For this review, take the finished solid that the model builds, in its own axes (mm). A direction names the side the tool comes from. Round coordinates to 2 decimals unless told otherwise and drop trailing zeros. Order: outer loops, then holes, each group sorted by start corner. A loop starts at its lowest first (then second) coordinate and runs counter-clockwise, first axis right, second up. Notation, with made-up numbers: M -33.5,-14.75 L 0.5,-14.75 A12 cw 0.5,2.25 Z; hole C 5.25,26.25 d7. An arc over 180 degrees is marked long. Answer as a JSON object with one key per item and string values.
from build123d import *

# Parameters (mm, degrees)
F0_W     = 12.7
F0_H     = 25.4
F1_DEPTH = 25.4
F3_DEPTH = 6.35
F5_D     = 6.35
F7_D     = 6.35


with BuildPart() as f1:
    # F0 (on Top) → F1 (new body)
    with BuildSketch(Plane.XY):
        with Locations((-6.35, 12.7)):
            Rectangle(F0_W, F0_H)
    extrude(amount=F1_DEPTH)

    # F2 (on Top) → F3 (join)
    with BuildSketch(Plane.XY):
        with BuildLine():
            Line((0, 25.4), (0, 0))
            Line((0, 0), (12.7, 0))
            ThreePointArc((12.7, 0), (25.4, 12.7), (12.7, 25.4))
            Line((12.7, 25.4), (0, 25.4))
        make_face()
    extrude(amount=F3_DEPTH)

    # F5 (through all)
    with Locations(Plane.YZ):
        with Locations((12.7, 15.875)):
            Hole(F5_D / 2)

    # F7 (through all)
    with Locations(Plane.XY.offset(6.35)):
        with Locations((12.7, 12.7)):
            Hole(F7_D / 2)


solid = f1.part
1) Add section B-B on x = -5. State the section outline as (y, z) points (3 decimals).
Geometry check:
{"outline": "M 0,0 L 25.4,0 L 25.4,25.4 L 0,25.4 Z; hole C 12.7,15.875 d6.35"}
2) Add section D-D on z = 15. State the section outline as (x, y) points.
Geometry check:
{"outline": "M -12.7,0 L 0,0 L 0,9.65 L -12.7,9.65 Z; M -12.7,15.75 L 0,15.75 L 0,25.4 L -12.7,25.4 Z"}
3) Add section C-C on z = 3.25. State the section outline as (x, y) points (3 decimals), and give its area (3 significant figures).
Geometry check:
{"outline": "M -12.7,0 L 12.7,0 A12.7 ccw 12.7,25.4 L -12.7,25.4 Z; hole C 12.7,12.7 d6.35", "area": "867 mm²"}
4) For L1, parallel to Z at x = -7.5, y = 12.7; L2, parallel to Y at x = 12.7, z = 2 (3 decimals); L3, parallel to X at y = 18, z = 24, list the stretches that pass through material, from the lowest coordinate up.
Geometry check:
{"L1": "z = 0 to 12.7, 19.05 to 25.4", "L2": "y = 0 to 9.525, 15.875 to 25.4", "L3": "x = -12.7 to 0"}
5) Mouldability with a two-part tool opening along Y and no side actions: class faces 3 (the cylindrical face through (-6.44, 9.67, 16.83)), 4 (the flat face through (-5, 25.4, 10)), 5 (the flat face through (6, 13, 0)) as +Y half, -Y half, draft (parallel to the pull), parting line (faces both ways), or undercut.
Geometry check:
{"face 3": "undercut", "face 4": "+Y half", "face 5": "draft"}
6) Insertion check: P1, Ø6, axis at y = 8.5, z = 14.5, coming from the +X side; P2, Ø4, axis at x = 12.7, y = 12.7, coming from the -Z side; P3, Ø4, axis at x = 10.5, y = 20, coming from the -Z side; P4, Ø2, axis at x = 6.5, y = 18, coming from the +Z side. Each pin has a flat end and moves straight along its axis. Give the tip position at first contact, or say it passes through.
Geometry check:
{"P1": "stops at x = 0", "P2": "passes through", "P3": "stops at z = 0", "P4": "stops at z = 6.35"}
7) Add section A-A on y = 12.7. State the section outline as (x, z) points (3 decimals).
Geometry check:
{"outline": "M -12.7,0 L 9.525,0 L 9.525,6.35 L 0,6.35 L 0,12.7 L -12.7,12.7 Z; M -12.7,19.05 L 0,19.05 L 0,25.4 L -12.7,25.4 Z; M 15.875,0 L 25.4,0 L 25.4,6.35 L 15.875,6.35 Z"}
8) Machinability: for faces 1 (the flat face through (-12.7, 12.5, 12.5)), 2 (the flat face through (10, 10, 6.35)), which of the approach directions +Z, -Z, +X, -X, +Y, -Y give a long, thin tool a straight path to every point of the face, cutting with its end or side? Answer none if there is none.
Geometry check:
{"face 1": "+Z, -Z, -X, +Y, -Y", "face 2": "+Z, +X, +Y, -Y"}
